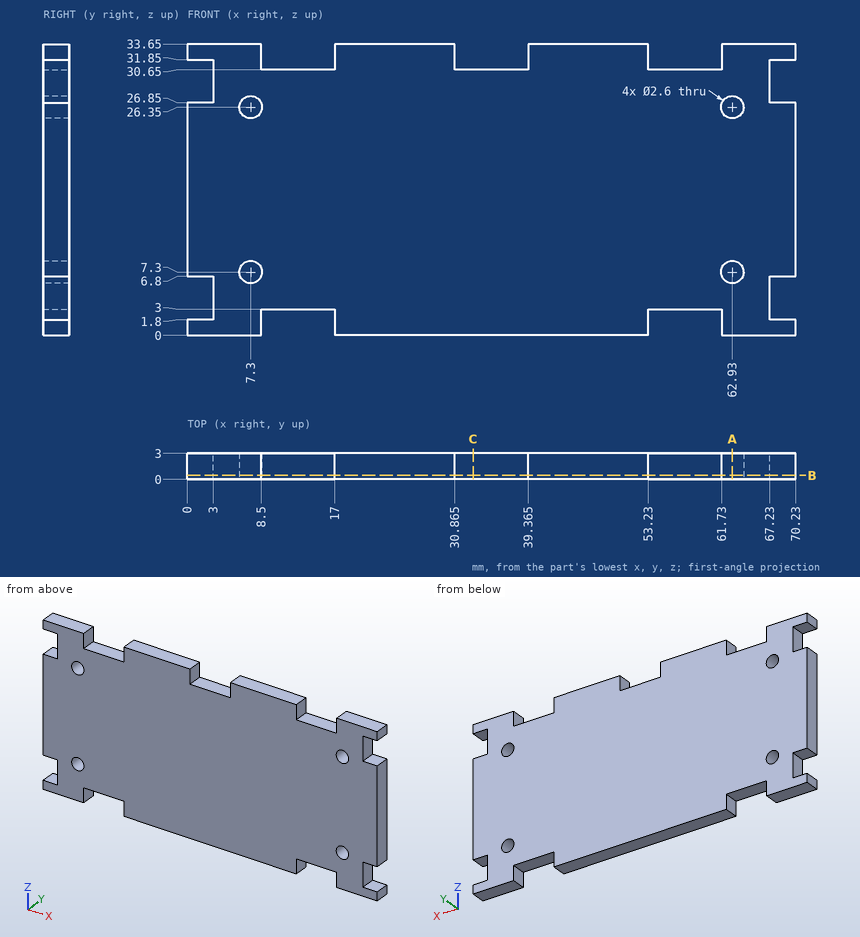
Check sheet for the drawn part. Datum: minimum x, y, z corner. Units: mm. Round coordinates to 2 decimals unless told otherwise and drop trailing zeros. Loops run counter-clockwise (first coordinate to the right, second up) from the corner with the lowest first, then second, coordinate; pieces in that order, holes last. Notation, with made-up numbers: (51, 10) - (93, 10) arc R19 ccw to (93, 42) - close; hole circle Ø5 at (49.5, 1). An arc over 180 degrees is marked (long way). Write item = value, one per line. Start each with the question number.
1. Section check A-A on x = 62.93. Enter the section's corners in (y, z), then the cut area to 4 significant figures.
2. Section check C-C on x = 33. Enter the section's corners in (y, z), then the cut area to 4 significant figures.
3. Depth check by flat-ended pin: pin 1 (0.9 mm diameter, centred on x = 37, y = 2, fed in from +Z); pin 2 (1.5 mm diameter, centred on x = 1.5, y = 2, fed in from -Z); pin 3 (1.5 mm diameter, centred on y = 2, z = 30, fed in from -X). Enter the tip coordinate at first touch or a pass-through.
4. Section check B-B on y = 0.45. Give the number of separate pieces and of enclosed holes in the cut face, then the cut area to 3 significant figures.
5. Thickness scan on line 1 (X direction, y = 1.7, z = 7.3); line 2 (Z direction, x = 8, y = 0.9); line 3 (X direction, y = 2.95, z = 7). Record the ranges inside material, lowest first.
Working result:
q1.outline = (0, 0) - (3, 0) - (3, 6) - (0, 6) - close; (0, 8.6) - (3, 8.6) - (3, 25.05) - (0, 25.05) - close; (0, 27.65) - (3, 27.65) - (3, 33.65) - (0, 33.65) - close
q1.area = 85.35 mm^2
q2.outline = (0, 0) - (3, 0) - (3, 30.65) - (0, 30.65) - close
q2.area = 91.95 mm^2
q3.pin_1 = 30.65
q3.pin_2 = 0
q3.pin_3 = 3
q4.separate_pieces = 1
q4.enclosed_holes = 4
q4.area = 2,150 mm^2
q5.line_1 = 0 to 6, 8.6 to 61.63, 64.23 to 70.23
q5.line_2 = 0 to 6.2, 8.4 to 25.25, 27.45 to 33.65
q5.line_3 = 0 to 6.04, 8.56 to 61.67, 64.19 to 70.23
